Part model, mm, in its own coordinate system. Face numbers are marked on the shaded views. Give positions to 0.01 mm unless a question says otherwise; leave off trailing zeros. Write each loop counter-clockwise with the first axis right and the second up, starting at its lowest first coordinate (ties: lowest second). Pieces come first, ordered by that corner, then holes. Notation, with made-up numbers: M 49.5,55.25 L 91.5,55.25 A25 cw 91.5,91.25 Z; hole C 56.25,4 d9. An arc over 180 degrees is marked long. Use a Markdown table: item, result.
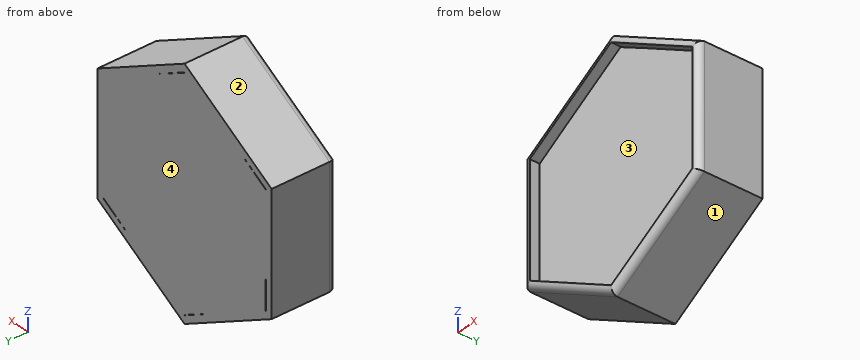
```python
from build123d import *

# Parameters (mm, degrees)
F1_DEPTH = 25.4
F3_DEPTH = 21.59
F4_R     = 2.54


with BuildPart() as f1:
    # F0 (on Front) → F1 (new body)
    with BuildSketch(Plane.XZ):
        Polygon((0.004891, 48.265907), (-41.797056, 24.137189), (-41.801947, -24.128718), (-0.004891, -48.265907), (41.797056, -24.137189), (41.801947, 24.128718), align=None)
        Polygon((-39.000372, 22.522145), (0.004563, 45.036386), (39.004936, 22.514241), (39.000372, -22.522145), (-0.004563, -45.036386), (-39.004936, -22.514241), align=None, mode=Mode.SUBTRACT)
    extrude(amount=F1_DEPTH)

    # F2 (on Front) → F3 (join)
    with BuildSketch(Plane.XZ):
        Polygon((38.877433, 22.890052), (-0.38465, 45.113871), (-39.262083, 22.223819), (-38.877433, -22.890052), (0.38465, -45.113871), (39.262083, -22.223819), align=None)
    extrude(amount=F3_DEPTH)

    # F4
    f4_edges = [f1.edges().sort_by_distance(p)[0] for p in [
        (-20.903419, -25.4, -36.197312),
        (-41.799501, -25.4, 0.004235),
        (-20.896083, -25.4, 36.201548),
        (20.896083, -25.4, -36.201548),
        (41.799501, -25.4, -0.004235),
        (20.903419, -25.4, 36.197312),
    ]]
    fillet(f4_edges, radius=F4_R)


solid = f1.part
```
1. Drop flat-ended pins along their axis: P1, Ø7, axis at y = -11.5, z = -8, coming from the +X side; P2, Ø10, axis at x = -20.5, y = -13, coming from the -Z side; P3, Ø8, axis at x = -25.5, y = -7.5, coming from the -Z side. Give the stop position or say it passes through.
Findings below:
| item | result |
|---|---|
| P1 | x = 41.8 |
| P2 | z = -39.32 |
| P3 | z = -35.85 |
2. Cut at A-A, the plane y = -7.75. Give the cut face in (x, z).
Findings below:
| item | result |
|---|---|
| outline | M -41.8,-24.13 L 0,-48.27 L 41.8,-24.14 L 41.8,24.13 L 0,48.27 L -41.8,24.14 Z; hole M -39,-22.51 L -38.88,-22.59 L -39,-8.11 Z; hole M -39,22.38 L -26.52,29.72 L -39,22.52 Z; hole M -12.48,-37.83 L 0,-45.04 L 0.12,-44.96 Z; hole M -0.12,44.96 L 12.48,37.83 L 0,45.04 Z; hole M 26.52,-29.72 L 39,-22.52 L 39,-22.38 Z; hole M 38.88,22.59 L 39,8.11 L 39,22.51 Z |
3. Two-plate mould, pull along Z, no slides. Class the marked faces 1, 2, 3 and 4: released by +Z, released by -Z, zero draft, split by the parting line, or undercut.
Findings below:
| item | result |
|---|---|
| face 1 | released by -Z |
| face 2 | released by +Z |
| face 3 | undercut |
| face 4 | zero draft |
4. Drill centre lines: L1, parallel to Y at x = 19, z = -10; L2, parallel to X at y = -3.5, z = 4; L3, parallel to X at y = -22, z = -38.5. Where is each one in solid material? Low to high.
Findings below:
| item | result |
|---|---|
| L1 | -21.59 to 0 |
| L2 | -41.8 to 41.8 |
| L3 | -16.92 to -11.32, 11.32 to 16.91 |
